Read the model definition and answer for the solid it produces. Units are mm, in the model's axes. A direction names the side the tool comes from. Give positions to 0.01 mm unless a question says otherwise; leave off trailing zeros. Write each loop counter-clockwise with the first axis right and the second up, starting at its lowest first coordinate (ties: lowest second). Pieces come first, ordered by that corner, then holes.
```python
from build123d import *

# Parameters (mm, degrees)
SKETCH1_R           = 2
BOSS_EXTRUDE1_DEPTH = 1.5


with BuildPart() as part:
    # Sketch1 → Boss-Extrude1 (new, symmetric)
    with BuildSketch(Plane(origin=(0, 0, 0), x_dir=(0, 0, -1), z_dir=(1, 0, 0))):
        with BuildLine():
            Line((0, 0), (0, 3))
            Line((0, 3), (25, 3))
            Line((25, 3), (25, 11))
            ThreePointArc((25, 11), (23.828427125, 13.828427125), (21, 15))
            Line((21, 15), (21, 8))
            Line((21, 8), (12, 8))
            Line((12, 8), (5, 15))
            Line((5, 15), (-11, 15))
            ThreePointArc((-11, 15), (-13.828427125, 13.828427125), (-15, 11))
            Line((-15, 11), (-15, 6))
            ThreePointArc((-15, 6), (-10.757359313, 4.242640687), (-9, 0))
            Line((-9, 0), (-9.002044324, -0.203364757))
            ThreePointArc((-9.002044324, -0.203364757), (-10.84433818, -4.409819928), (-15.121449634, -6.081534426))
            Line((-15.121449634, -6.081534426), (-15.221964484, -11.080524))
            ThreePointArc((-15.221964484, -11.080524), (-14.107488152, -13.931931636), (-11.303184704, -15.16012754))
            Line((-11.303184704, -15.16012754), (4.693581934, -15.48177506))
            Line((4.693581934, -15.48177506), (11.832888128, -8.623910446))
            Line((11.832888128, -8.623910446), (20.831069362, -8.804837176))
            Line((20.831069362, -8.804837176), (20.690348572, -15.80342258))
            ThreePointArc((20.690348572, -15.80342258), (23.541756208, -14.688946248), (24.769952111, -11.884642801))
            Line((24.769952111, -11.884642801), (24.930775871, -3.886259482))
            Line((24.930775871, -3.886259482), (-0.064172001, -3.383685231))
            Line((-0.064172001, -3.383685231), (-0.00386309, -0.384291487))
            Line((-0.00386309, -0.384291487), (0, 0))
        make_face()
        with Locations((-11, 11)):
            Circle(SKETCH1_R, mode=Mode.SUBTRACT)
        with Locations(Location((-11.222772824, -11.16093588, 0), (0, 0, 180))):
            Circle(SKETCH1_R, mode=Mode.SUBTRACT)
    extrude(amount=BOSS_EXTRUDE1_DEPTH, both=True)


solid = part.part
```
Item 1: Which of the six approach directions +Z, -Z, +X, -X, +Y, -Y give full straight-line access (tool end or side, diameter ignored) to faces 1 (the flat face through (0, 8, -17)), 2 (the flat face through (1.5, 3.2, -4.6)), 3 (the flat face through (0.021, -12.101, -8.213)), 4 (the flat face through (-1.5, 3.2, -4.6)), 5 (the flat face through (0, 3, -12))?
Result set:
face 1: +X, -X, +Y
face 2: +Z, -Z, +X, +Y, -Y
face 3: +X, -X, -Y
face 4: +Z, -Z, -X, +Y, -Y
face 5: -Z, +X, -X
Item 2: Section C-C (y = 10.5) is taken. Write down the section's boundary in (x, z), and give its area (3 significant figures).
Result set:
outline: (-1.5, -25) - (1.5, -25) - (1.5, -21) - (-1.5, -21) - close; (-1.5, -9.5) - (1.5, -9.5) - (1.5, 9.06) - (-1.5, 9.06) - close; (-1.5, 12.94) - (1.5, 12.94) - (1.5, 15) - (-1.5, 15) - close
area: 73.9 mm2
Item 3: Determine the mould class of faces 6 (the flat face through (0, 9, 15)), 7 (the cylindrical face through (0.02, -14.72, -23.51)), 8 (the flat face through (0, 1, 0)), 9 (the cylindrical face through (0.021, -4.364, 10.797)) for opening direction Y: pulls with the +Y half, pulls with the -Y half, needs draft (parallel to the pull), parting line crosses it, or undercut.
Result set:
face 6: needs draft
face 7: pulls with the -Y half
face 8: undercut
face 9: undercut
Item 4: Find the intervals of material crossed by line 1 along Z through (x, y) = (0.5, 11.5); line 2 along Z through (x, y) = (1.3, -12); line 3 along Y through (x, z) = (-0.6, 11), in increasing order.
Result set:
line 1: z = -24.97 to -21, -8.5 to 9.06, 12.94 to 14.97
line 2: z = -24.77 to -20.77, -8.32 to 9.41, 13.04 to 15.13
line 3: y = -15.17 to -13.15, -9.17 to -4.55, 4.47 to 9, 13 to 15
Item 5: Section A-A (z = -14) is taken. Write down the section's boundary in (x, y), and give its area (3 significant figures).
Result set:
outline: (-1.5, -8.67) - (1.5, -8.67) - (1.5, -3.67) - (-1.5, -3.67) - close; (-1.5, 3) - (1.5, 3) - (1.5, 8) - (-1.5, 8) - close
area: 30.0 mm2
Item 6: Each of these flat-tipped pins is pushed along its axis until it touches: pin 1 Ø1.5 at (x, z) = (-1, -8.5) entering from +Y; pin 2 Ø1.5 at (x, y) = (0.5, 9) entering from +Z; pin 3 Ø3 at (y, z) = (-11.16, 11.22) entering from +X; pin 4 Ø0.9 at (x, z) = (-0.5, -17) entering from +Y. Where does it stop, or does it pass through?
Result set:
pin 1: stops at y = 12.25
pin 2: stops at z = 15
pin 3: passes through
pin 4: stops at y = 8
Item 7: Section B-B (z = 10) is taken. Write down the section's boundary in (x, y), and give its area (3 significant figures).
Result set:
outline: (-1.5, -15.19) - (1.5, -15.19) - (1.5, -12.74) - (-1.5, -12.74) - close; (-1.5, -9.58) - (1.5, -9.58) - (1.5, -3.4) - (-1.5, -3.4) - close; (-1.5, 3.32) - (1.5, 3.32) - (1.5, 9.27) - (-1.5, 9.27) - close; (-1.5, 12.73) - (1.5, 12.73) - (1.5, 15) - (-1.5, 15) - close
area: 50.5 mm2
Item 8: Section D-D (x = 0.45) is taken. Write down the section's boundary in (y, z), and give its area (3 significant figures).
Result set:
outline: (-15.8, -20.69) arc R4 ccw to (-11.88, -24.77) - (-3.89, -24.93) - (-3.38, 0.06) - (-0.38, 0) - (0, 0) - (3, 0) - (3, -25) - (11, -25) arc R4 ccw to (15, -21) - (8, -21) - (8, -12) - (15, -5) - (15, 11) arc R4 ccw to (11, 15) - (6, 15) arc R6 cw to (0, 9) - (-0.2, 9) arc R6 cw to (-6.08, 15.12) - (-11.08, 15.22) arc R4 ccw to (-15.16, 11.3) - (-15.48, -4.69) - (-8.62, -11.83) - (-8.8, -20.83) - close; hole circle Ø4 at (-11.16, 11.22); hole circle Ø4 at (11, 11)
area: 782 mm2
